Verification items for the finished model (mm, model axes). A direction names the side the tool comes from. Give positions to 0.01 mm unless a question says otherwise; leave off trailing zeros. Loops run counter-clockwise (first coordinate to the right, second up) from the corner with the lowest first, then second, coordinate; pieces in that order, holes last. Notation, with made-up numbers: (-5.75, -12.75) - (48.25, -12.75) arc R12 ccw to (48.25, 10.25) - close; hole circle Ø11 at (41.25, 11). An arc over 180 degrees is marked (long way). Answer in a Markdown table with one row per item.
```python
from build123d import *

# Parameters (mm, degrees)
EXTRUDE_2_DEPTH     = 10
SKETCH_3_R          = 1.5
EXTRUDE_3_DEPTH     = 1.5
SKETCH_5_R          = 1.65
CUT_EXTRUDE_2_DEPTH = 27.084669827
FILLET_1_R          = 6
SKETCH_6_W          = 10
SKETCH_6_H          = 1
SKETCH_6_W_2        = 5
EXTRUDE_4_DEPTH     = 4
SKETCH_7_W          = 5.689599517
SKETCH_7_H          = 3.3
CUT_EXTRUDE_3_DEPTH = 0.5
SKETCH_8_W          = 11.306526487
SKETCH_8_H          = 19.042570926
CUT_EXTRUDE_4_DEPTH = 30.624989451
MOVE_FACE_1_BY      = 12
CUT_EXTRUDE_5_REACH = 31.625
SKETCH_9_W          = 14.188350819
SKETCH_9_H          = 12
SKETCH_10_R         = 1.65
CUT_EXTRUDE_6_DEPTH = 30.302559615
FILLET_2_R          = 6
MOVE_FACE_2_BY      = 1
FILLET_3_R          = 1


with BuildPart() as part:
    # Эскиз2 → Бобышка-Вытянуть2 (new body)
    with BuildSketch(Plane.XY):
        Polygon((0, 0), (0, 2), (13, 2), (13, -0.1), (24, -0.1), (24, -2.1), (11, -2.1), (11, 0), align=None)
    extrude(amount=EXTRUDE_2_DEPTH)

    # Эскиз3 → Бобышка-Вытянуть3 (add)
    with BuildSketch(Plane(origin=(0, -0.1, 0), x_dir=(1, 0, 0), z_dir=(0, 1, 0))):
        with Locations(Location((18.1, -5, 0), (0, 0, 90))):
            Circle(SKETCH_3_R)
    extrude(amount=EXTRUDE_3_DEPTH)

    # Эскиз5 → Вырез-Вытянуть2 (cut, through all)
    with BuildSketch(Plane.XZ):
        with Locations((5, 5)):
            Circle(SKETCH_5_R)
    extrude(amount=-CUT_EXTRUDE_2_DEPTH, mode=Mode.SUBTRACT)

    # Скругление1
    fillet_1_edges = [part.edges().sort_by_distance(p)[0] for p in [
        (24, -1.1, 10),
        (0, 1, 10),
    ]]
    fillet(fillet_1_edges, radius=FILLET_1_R)

    # Эскиз6 → Бобышка-Вытянуть4 (add)
    with BuildSketch(Plane(origin=(0, -2.1, 0), x_dir=(-1, 0, 0), z_dir=(0, -1, 0))):
        with Locations((-16, -0.5)):
            Rectangle(SKETCH_6_W, SKETCH_6_H)
        with Locations((-13.5, -9.5)):
            Rectangle(SKETCH_6_W_2, SKETCH_6_H)
    extrude(amount=EXTRUDE_4_DEPTH)

    # Эскиз7 → Вырез-Вытянуть3 (cut)
    with BuildSketch(Plane.XZ):
        with Locations((2.155200242, 5)):
            Rectangle(SKETCH_7_W, SKETCH_7_H)
    extrude(amount=-CUT_EXTRUDE_3_DEPTH, mode=Mode.SUBTRACT)

    # Зеркальное отражение1: part across plane


with BuildPart() as part_1:
    add(part.part)
    add(part.part.mirror(Plane.ZX.offset(-6.1)))

    # Эскиз8 → Вырез-Вытянуть4 (cut, through all)
    with BuildSketch(Plane.XY.offset(10)):
        with Locations((5.346736757, -6.608790605)):
            Rectangle(SKETCH_8_W, SKETCH_8_H)
    extrude(amount=-CUT_EXTRUDE_4_DEPTH, mode=Mode.SUBTRACT)

    # Move Face 1: a face moved outward by 12.0
    extrude(part_1.faces().sort_by_distance((11, -10.15, 5))[0], amount=MOVE_FACE_1_BY, dir=(-1, 0, 0))

    # Вырез-Вытянуть5: up to this face of the body (flat: up to its plane)
    cut_extrude_5_end = Plane(part_1.part.faces().sort_by_distance((10, -6.1, 1))[0])
    # Эскиз9 → Вырез-Вытянуть5 (cut, up to the picked face)
    with BuildSketch(Plane.XY.offset(10), mode=Mode.PRIVATE) as cut_extrude_5_sk1:
        with Locations((3.90582459, -6.1)):
            Rectangle(SKETCH_9_W, SKETCH_9_H)
    cut_extrude_5_tool1 = split(extrude(cut_extrude_5_sk1.sketch, amount=-CUT_EXTRUDE_5_REACH, mode=Mode.PRIVATE), bisect_by=cut_extrude_5_end, keep=Keep.BOTH, mode=Mode.PRIVATE)
    add(cut_extrude_5_tool1.solids().sort_by(Axis((3.905825, -6.1, 10), (0, 0, -1)))[0], mode=Mode.SUBTRACT)

    # Эскиз10 → Вырез-Вытянуть6 (cut, through all)
    with BuildSketch(Plane.XY.offset(1)):
        with Locations((2, -9.1)):
            Circle(SKETCH_10_R)
        with Locations((8, -3.1)):
            Circle(SKETCH_10_R)
    extrude(amount=-CUT_EXTRUDE_6_DEPTH, mode=Mode.SUBTRACT)

    # Скругление2
    fillet_2_edges = [part_1.edges().sort_by_distance(p)[0] for p in [
        (-1, -13.15, 10),
        (-1, 0.95, 10),
    ]]
    fillet(fillet_2_edges, radius=FILLET_2_R)

    # Move Face 2: a face moved outward by 1.0
    extrude(part_1.faces().sort_by_distance((9.253385216, -6.1, 1))[0], amount=MOVE_FACE_2_BY, dir=(0, 0, 1))

    # Скругление3
    fillet_3_edges = [part_1.edges().sort_by_distance(p)[0] for p in [
        (21, -6.1, 2),
    ]]
    fillet(fillet_3_edges, radius=FILLET_3_R)


solid = part_1.part
```
Q1. Sectioned sample at A-A (y = -5.25). Record the cut outline in (x, z), and give its area (3 significant figures).
Completed:
| item | result |
|---|---|
| outline | (-1, 0) - (21, 0) - (21, 1) arc R1 ccw to (20, 2) - (-1, 2) - close; (11, 9) - (16, 9) - (16, 10) - (11, 10) - close |
| area | 48.8 mm^2 |
Q2. Go/stop test with flat-tipped pins: P1, Ø3, axis at x = 15, z = 7, coming from the -Y side; P2, Ø5.5, axis at x = 2, y = -9.1, coming from the +Z side; P3, Ø3.5, axis at x = 18.5, z = 5.5, coming from the +Y side. Record where each tip stops, or that it passes through.
Completed:
| item | result |
|---|---|
| P1 | y = -12.1 |
| P2 | z = 2 |
| P3 | y = 1.4 |
Q3. Sectioned sample at C-C (y = -3.1). Record the cut outline in (x, z), and give its area (3 significant figures).
Completed:
| item | result |
|---|---|
| outline | (-1, 0) - (6.35, 0) - (6.35, 2) - (-1, 2) - close; (9.65, 0) - (21, 0) - (21, 1) arc R1 ccw to (20, 2) - (9.65, 2) - close; (11, 9) - (16, 9) - (16, 10) - (11, 10) - close |
| area | 42.2 mm^2 |
Q4. Draft check along X on faces 1 (the face through (16, -6.2, 9.5)), 2 (the face through (6, 2, 5)), 3 (the face through (16.613, -12.84, 5.195)). Enter one of: +X half, -X half, draft (parallel to the pull), parting line (faces both ways), or undercut.
Completed:
| item | result |
|---|---|
| face 1 | +X half |
| face 2 | draft |
| face 3 | undercut |
Q5. Thickness scan on line 1 (Z direction, x = 11.25, y = -3); line 2 (Y direction, x = 10.5, z = 2.75); line 3 (Y direction, x = 19, z = 5). Record the ranges inside material, lowest first.
Completed:
| item | result |
|---|---|
| line 1 | 0 to 2, 9 to 10 |
| line 2 | -14.2 to -12.1, -0.1 to 2 |
| line 3 | -13.6 to -10.1, -2.1 to 1.4 |
Q6. Sectioned sample at D-D (z = 4.5). Record the cut outline in (x, y), and give its area (3 significant figures).
Completed:
| item | result |
|---|---|
| outline | (-0.98, -14.2) - (13, -14.2) - (13, -12.1) - (16.69, -12.1) - (16.69, -13.6) - (19.51, -13.6) - (19.51, -12.1) - (23.98, -12.1) - (23.98, -10.1) - (11, -10.1) - (11, -12.1) - (-0.98, -12.1) - close; (-0.98, -0.1) - (11, -0.1) - (11, -2.1) - (23.98, -2.1) - (23.98, -0.1) - (19.51, -0.1) - (19.51, 1.4) - (16.69, 1.4) - (16.69, -0.1) - (13, -0.1) - (13, 2) - (-0.98, 2) - close |
| area | 119 mm^2 |
Q7. Tool access check on faces 4 (the face through (13, 1, 5)), 5 (the face through (18, -13.6, 5)), 6 (the face through (18, -10.1, 5)). Record the directions out of +Z, -Z, +X, -X, +Y, -Y that give a thin tool (end or side, any length) a straight path to the whole face; none if there is none.
Completed:
| item | result |
|---|---|
| face 4 | +Z, -Z, +Y |
| face 5 | +Z, -Z, +X, -Y |
| face 6 | +X |
Q8. Sectioned sample at B-B (x = 13.75). Record the cut outline in (y, z), and give its area (3 significant figures).
Completed:
| item | result |
|---|---|
| outline | (-12.1, 0) - (-0.1, 0) - (-0.1, 10) - (-12.1, 10) - close; hole (-10.1, 2) - (-2.1, 2) - (-2.1, 9) - (-10.1, 9) - close |
| area | 64.0 mm^2 |
